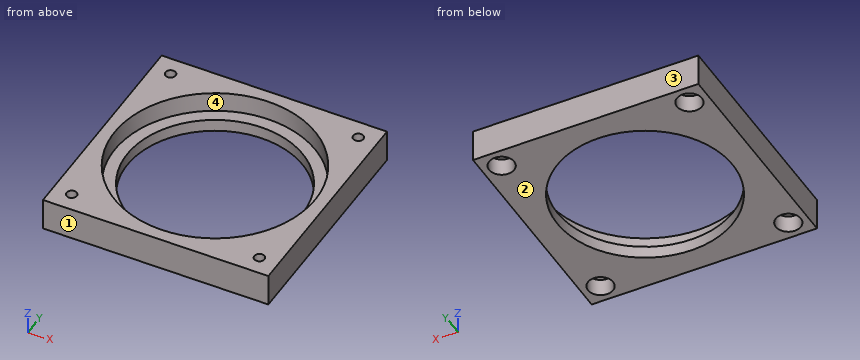
Autodesk Inventor part; units mm, degrees
ref_plane "YZ Plane" through (0, 0, 0) normal (1, 0, 0) x (0, 1, 0)
ref_plane "XZ Plane" through (0, 0, 0) normal (0, 1, 0) x (-1, 0, 0)
ref_plane "XY Plane" through (0, 0, 0) normal (0, 0, 1) x (1, 0, 0)
sketch "Sketch4" plane through (0, 0, 0) normal (0, 0, 1) x (1, 0, 0)
  line L0 (-45, -45) -> (45, -45)
  line L1 (45, -45) -> (45, 45)
  line L2 (45, 45) -> (-45, 45)
  line L3 (-45, 45) -> (-45, -45)
  line L4 (-45, -45) -> (45, 45) construction
  line L5 (45, -45) -> (-45, 45) construction
  point P0 (0, 0)
  dimension "d10" = 90
  dimension "d11" = 90
extrude "Extrusion4" add sketch "Sketch4" along normal blind 5
sketch "Sketch5" plane through (0, 0, 5) normal (0, 0, 1) x (1, 0, 0)
  line L0 (-45, -45) -> (45, -45)
  line L1 (45, -45) -> (45, 45)
  line L2 (45, 45) -> (-45, 45)
  line L3 (-45, 45) -> (-45, -45)
  line L4 (-45, -45) -> (45, 45) construction
  line L5 (45, -45) -> (-45, 45) construction
  line L6 (45, 45) -> (-45, 45)
  line L7 (45, -45) -> (45, 45)
  circle A0 centre (0, 0) radius 40.05
  dimension "d14" = 80.1
extrude "Extrusion5" add sketch "Sketch5" along normal blind 8.1
sketch "Sketch6" plane through (0, 0, 5) normal (0, 0, 1) x (1, 0, 0)
  circle A0 centre (0, 0) radius 35
  dimension "d17" = 70
extrude "Extrusion6" cut sketch "Sketch6" against normal through all
sketch "Sketch7" plane through (0, 0, 0) normal (0, 0, -1) x (-1, 0, 0)
  circle A0 centre (-37.5, -37.5) radius 2.05
  circle A1 centre (-37.5, 37.5) radius 2.05
  circle A2 centre (37.5, 37.5) radius 2.05
  circle A3 centre (37.5, -37.5) radius 2.05
  line L0 (-45, -45) -> (-45, 45)
  line L1 (45, -45) -> (-45, -45)
  line L2 (-45, 45) -> (45, 45)
  line L3 (45, 45) -> (45, -45)
  point P0 (0, 0)
  dimension "d20" = 4.1
  dimension "d21" = 4.1
  dimension "d22" = 4.1
  dimension "d23" = 4.1
  dimension "d24" = 7.5
  dimension "d25" = 7.5
  dimension "d26" = 7.5
  dimension "d27" = 7.5
  dimension "d28" = 7.5
  dimension "d29" = 7.5
  dimension "d30" = 7.5
  dimension "d31" = 7.5
extrude "Extrusion7" cut sketch "Sketch7" against normal through all contours A0 | A1 | A2 | A3
sketch "Sketch8" plane through (0, 0, 0) normal (0, 0, -1) x (-1, 0, 0)
  circle A0 centre (-37.5, -37.5) radius 2.05
  circle A1 centre (-37.5, 37.5) radius 2.05
  circle A2 centre (37.5, 37.5) radius 2.05
  circle A3 centre (37.5, -37.5) radius 2.05
  circle A4 centre (-37.5, -37.5) radius 5
  circle A5 centre (-37.5, 37.5) radius 5
  circle A6 centre (37.5, 37.5) radius 5
  circle A7 centre (37.5, -37.5) radius 5
  point P0 (0, 0)
  dimension "d34" = 10
  dimension "d35" = 10
  dimension "d36" = 10
  dimension "d37" = 10
extrude "Extrusion8" cut sketch "Sketch8" against normal blind 7 contours A1 | A2 | A4 | A5 | A6 | A7
properties part number "bearing_bracket1" material "ABS Plastic"
Source: CAD feature listing. Evaluate the final solid. Frame: model axes, mm. Face numbers are marked on the shaded views. Coordinates: 2 decimals unless noted, no trailing zeros. Loops run counter-clockwise (first coordinate to the right, second up) from the corner with the lowest first, then second, coordinate; pieces in that order, holes last. Notation, with made-up numbers: (-20.75, -4) - (-1.75, -4) arc R22 ccw to (-1.75, 5) - close; hole circle Ø7 at (6.25, 58.25). An arc over 180 degrees is marked (long way). Answer as CSV lines item,"result".
1. Section C-C (y = 2). Return loops of the section in (x, z).
Established:
outline,"(-45, 0) - (-34.94, 0) - (-34.94, 5) - (-40, 5) - (-40, 13.1) - (-45, 13.1) - close; (34.94, 0) - (45, 0) - (45, 13.1) - (40, 13.1) - (40, 5) - (34.94, 5) - close"
2. Section B-B (z = 8.5). Return loops of the section in (x, y), then the cut area to 3 significant figures.
Established:
outline,"(-45, -45) - (45, -45) - (45, 45) - (-45, 45) - close; hole circle Ø80.1 at (0, 0); hole circle Ø4.1 at (-37.5, -37.5); hole circle Ø4.1 at (-37.5, 37.5); hole circle Ø4.1 at (37.5, -37.5); hole circle Ø4.1 at (37.5, 37.5)"
area,"3,010 mm2"
3. Mould query, pull axis Y, two halves, no side actions, for the marked faces 1, 2, 3 and 4. Classes: released by +Y, released by -Y, zero draft, split by the parting line, or undercut.
Established:
face 1,"released by -Y"
face 2,"zero draft"
face 3,"released by +Y"
face 4,"undercut"
4. Section D-D (z = 2.5). Return loops of the section in (x, y), then the cut area to 3 significant figures.
Established:
outline,"(-45, -45) - (45, -45) - (45, 45) - (-45, 45) - close; hole circle Ø10 at (-37.5, -37.5); hole circle Ø10 at (-37.5, 37.5); hole circle Ø70 at (0, 0); hole circle Ø10 at (37.5, -37.5); hole circle Ø10 at (37.5, 37.5)"
area,"3,940 mm2"
5. Section A-A (x = 0). Return loops of the section in (y, z).
Established:
outline,"(-45, 0) - (-35, 0) - (-35, 5) - (-40.05, 5) - (-40.05, 13.1) - (-45, 13.1) - close; (35, 0) - (45, 0) - (45, 13.1) - (40.05, 13.1) - (40.05, 5) - (35, 5) - close"
6. Ray query, line 1 (Y direction, x = -37.5, z = 2.25); line 2 (Z direction, x = -38, y = -34); line 3 (X direction, y = 29, z = 11.75). Return the intervals inside material, ascending.
Established:
line 1,"y = -45 to -42.5, -32.5 to 32.5, 42.5 to 45"
line 2,"z = 7 to 13.1"
line 3,"x = -45 to -27.62, 27.62 to 45"
7. Contact query for a flat-ended pin moving along its axis: pin 1 (5.5 mm diameter, centred on x = 37.5, y = 37.5, fed in from -Z). Output: stop coordinate, or through.
Established:
pin 1,"stops at z = 7"
